Autodesk Inventor part; units mm, degrees
ref_plane "YZ Plane" through (0, 0, 0) normal (1, 0, 0) x (0, 1, 0)
ref_plane "XZ Plane" through (0, 0, 0) normal (0, 1, 0) x (-1, 0, 0)
ref_plane "XY Plane" through (0, 0, 0) normal (0, 0, 1) x (1, 0, 0)
sketch "Sketch1" plane through (0, 0, 0) normal (0, 1, 0) x (-1, 0, 0)
  circle A0 centre (0, 0) radius 8.75
  circle A1 centre (0, 0) radius 6.25
  dimension "d0" = 17.5
  dimension "d1" = 12.5
extrude "Extrusion1" add sketch "Sketch1" along normal blind 3.3
sketch "Sketch2" plane through (0, 3.3, 0) normal (0, 1, 0) x (1, 0, 0)
  circle A0 centre (0, 0) radius 8.75
  line L0 (-4.9722, -7.2) -> (4.9722, -7.2)
  line L1 (4.9722, 7.2) -> (-4.9722, 7.2)
  line L2 (-12.7989, 0) -> (12.7989, 0) construction
  dimension "d4" = 14.4
extrude "Extrusion2" cut sketch "Sketch2" against normal blind 1 contours A0 L0 L1
properties part number "Toggle_Collar" material "PC/ABS Plastic"
Geometry check sheet. Reference: the model listing, model coordinates, mm. A direction names the side the tool comes from. Round coordinates to 2 decimals unless told otherwise and drop trailing zeros. Loops run counter-clockwise (first coordinate to the right, second up) from the corner with the lowest first, then second, coordinate; pieces in that order, holes last.
Item 1: Access from +Z, -Z, +X, -X, +Y, -Y to the whole of each face (thin tool, end or side, straight path). Record for faces 4 (the flat face through (0, 3.3, 8)), 5 (the flat face through (0, 3, -7.2)).
Item 2: Cross-section at C-C on y = 1.55. Record the boundary of the cut face in (x, z).
Item 3: Gauge pin test, flat ends, axial feed: pin 1 (7 mm diameter, centred on x = 2, z = -1.5, fed in from +Y); pin 2 (0.5 mm diameter, centred on x = -0.5, y = 3, fed in from +Z); pin 3 (4 mm diameter, centred on x = -5.5, z = -2.5, fed in from +Y). Record the tip position at first contact, or that the pin passes through.
Item 4: Cross-section at B-B on x = 0. Record the boundary of the cut face in (y, z), then the cut area to 3 significant figures.
Item 5: Mould release check, pull along Z, two halves, no side actions. Record for faces 1 (the flat face through (0, 3, 7.2)), 2 (the cylindrical face through (-8.083, 1.26, 3.351)), 3 (the flat face through (-6, 0, -4)): pulls with the +Z half, pulls with the -Z half, needs draft (parallel to the pull), parting line crosses it, or undercut.
Item 6: Cross-section at A-A on z = 0. Record the boundary of the cut face in (x, y), then the cut area to 3 significant figures.
Item 7: Thickness scan on line 1 (Z direction, x = 0, y = 0.9); line 2 (Y direction, x = -5.5, z = 5.25). Record the ranges inside material, lowest first.
Item 8: Cross-section at D-D on x = 7. Record the boundary of the cut face in (y, z).
Answer sheet:
1. face 4: +Z, -Z, +X, -X, +Y
1. face 5: +X, -X, +Y
2. outline: circle Ø17.5 at (0, 0); hole circle Ø12.5 at (0, 0)
3. pin 1: passes through
3. pin 2: stops at z = 8.75
3. pin 3: stops at y = 2.3
4. outline: (0, -8.75) - (3.3, -8.75) - (3.3, -7.2) - (2.3, -7.2) - (2.3, -6.25) - (0, -6.25) - close; (0, 6.25) - (2.3, 6.25) - (2.3, 7.2) - (3.3, 7.2) - (3.3, 8.75) - (0, 8.75) - close
4. area: 14.6 mm2
5. face 1: undercut
5. face 2: parting line crosses it
5. face 3: needs draft
6. outline: (-8.75, 0) - (-6.25, 0) - (-6.25, 2.3) - (-8.75, 2.3) - close; (6.25, 0) - (8.75, 0) - (8.75, 2.3) - (6.25, 2.3) - close
6. area: 11.5 mm2
7. line 1: z = -8.75 to -6.25, 6.25 to 8.75
7. line 2: y = 0 to 2.3
8. outline: (0, -5.25) - (2.3, -5.25) - (2.3, 5.25) - (0, 5.25) - close
